```python
from build123d import *

# Parameters (mm, degrees)
ESBO_O1_W                                    = 22.4
ESBO_O1_H                                    = 15
RESSALTO_EXTRUS_O1_DEPTH                     = 2
ESBO_O9_W                                    = 2
ESBO_O9_H                                    = 15
RESSALTO_EXTRUS_O2_DEPTH                     = 1
INCLINA_O2_ANGLE                             = 45
ESBO_O11_W                                   = 2
ESBO_O11_H                                   = 21.213203436
RESSALTO_EXTRUS_O4_DEPTH                     = 22
FILETE1_START                                = 20.4
FILETE1_DEPTH                                = 2
FILETE1_2_DEPTH                              = 22.4
FILETE1_3_DEPTH                              = 2
ESCAREADO_PARA_SFHCS_M31_D                   = 3.4
ESCAREADO_PARA_SFHCS_M31_DEPTH               = 7.5
ESCAREADO_PARA_SFHCS_M31_CSINK_D             = 6.72
ESCAREADO_PARA_SFHCS_M31_CSINK_ANGLE         = 90
ESCAREADO_PARA_SFHCS_M31_TIP                 = 1.021463052
FILETE2_R                                    = 3
ESCAREADO_PARA_PARAFUSO_COM_CABE_A_E_2_COUNT = 2
ESCAREADO_PARA_PARAFUSO_COM_CABE_A_E_2_PITCH = 9


with BuildPart() as part:
    # Esboço1 → Ressalto-extrusão1 (new body)
    with BuildSketch(Plane(origin=(0, 0, 0), x_dir=(1, 0, 0), z_dir=(0, 1, 0))):
        with Locations((11.2, 7.5)):
            Rectangle(ESBO_O1_W, ESBO_O1_H)
    extrude(amount=RESSALTO_EXTRUS_O1_DEPTH)

    # Esboço9 → Ressalto-extrusão2 (add)
    with BuildSketch(Plane.XZ):
        with Locations((21.4, -7.5)):
            Rectangle(ESBO_O9_W, ESBO_O9_H)
    extrude(amount=RESSALTO_EXTRUS_O2_DEPTH)

    # Inclinação2
    inclina_o2_faces = [part.faces().sort_by_distance(p)[0] for p in [
        (21.4, -1, -7.5),
    ]]
    draft(inclina_o2_faces, Plane(origin=(0, 2, 0), x_dir=(1, 0, 0), z_dir=(0, 0, 1)), INCLINA_O2_ANGLE)

    # Esboço11 → Ressalto-extrusão4 (add)
    with BuildSketch(Plane(origin=(0, -0.5, 0.5), x_dir=(1, 0, 0), z_dir=(0, -0.7071067811865462, 0.7071067811865488))):
        with Locations((21.4, -11.313708499)):
            Rectangle(ESBO_O11_W, ESBO_O11_H)
    extrude(amount=RESSALTO_EXTRUS_O4_DEPTH)

    # Filete1: read off the stored shape, not the designer's step
    # Filete1 outline → Filete1 (cut)
    with BuildSketch(Plane.YZ.offset(FILETE1_START)):
        with BuildLine():
            ThreePointArc((-23.627416998, 8.485281374), (-16.556349186, 11.414213562), (-9.485281374, 8.485281374))
            Line((-9.485281374, 8.485281374), (-16.556349186, 15.556349186))
            Line((-16.556349186, 15.556349186), (-23.627416998, 8.485281374))
        make_face()
        with BuildLine():
            Line((-16, -15), (-11.857864376, -15))
            ThreePointArc((-11.857864376, -15), (-15.6846987, -14.238795325), (-18.928932188, -12.071067812))
            Line((-18.928932188, -12.071067812), (-16, -15))
        make_face()
        with BuildLine():
            ThreePointArc((-24.485281374, -6.514718626), (-27.414213562, 0.556349186), (-24.485281374, 7.627416998))
            Line((-24.485281374, 7.627416998), (-31.556349186, 0.556349186))
            Line((-31.556349186, 0.556349186), (-24.485281374, -6.514718626))
        make_face()
    extrude(amount=FILETE1_DEPTH, mode=Mode.SUBTRACT)

    # Filete1 2 outline → Filete1 2 (add)
    with BuildSketch(Plane.YZ):
        with BuildLine():
            Line((0, 0), (2, 0))
            ThreePointArc((2, 0), (0.988246282, 0.177135355), (0, 0.457120724))
            Line((0, 0.457120724), (0, 0))
        make_face()
    extrude(amount=FILETE1_2_DEPTH)

    # Filete1 3 outline → Filete1 3 (add)
    with BuildSketch(Plane.YZ.offset(FILETE1_START)):
        with BuildLine():
            Line((0, 0), (0, 0.457120724))
            ThreePointArc((0, 0.457120724), (-2.065182242, 1.434278965), (-3.854676043, 2.854676043))
            Line((-3.854676043, 2.854676043), (-1, 0))
            Line((-1, 0), (0, 0))
        make_face()
    extrude(amount=FILETE1_3_DEPTH)

    # Escareado para SFHCS M31
    with Locations(Plane(origin=(22.4, 0, 0), x_dir=(0, 0, -1), z_dir=(1, 0, 0))):
        with Locations((3, -6), (11, -14), (3, -22), (-5, -14)):
            CounterSinkHole(ESCAREADO_PARA_SFHCS_M31_D / 2, ESCAREADO_PARA_SFHCS_M31_CSINK_D / 2, depth=ESCAREADO_PARA_SFHCS_M31_DEPTH, counter_sink_angle=ESCAREADO_PARA_SFHCS_M31_CSINK_ANGLE)
            with Locations((0, 0, -(ESCAREADO_PARA_SFHCS_M31_DEPTH + ESCAREADO_PARA_SFHCS_M31_TIP / 2))):  # 118° drill point
                Cone(0, ESCAREADO_PARA_SFHCS_M31_D / 2, ESCAREADO_PARA_SFHCS_M31_TIP, mode=Mode.SUBTRACT)

    # Filete2
    # the kernel refuses this fillet: 3 mm, written as the material it adds along each edge
    with BuildSketch(Plane(origin=(20.4, 0, -15), x_dir=(-1, 0, 0), z_dir=(0, 0, 1))) as filete2_piece_1_section:
        with BuildLine():
            CenterArc((FILETE2_R, FILETE2_R), FILETE2_R, 180, 90)
            Line((0, FILETE2_R), (0, 0))
            Line((0, 0), (FILETE2_R, 0))
        make_face()
    filete2_piece_1 = extrude(amount=22.957120724, mode=Mode.PRIVATE)
    filete2_piece_1 = filete2_piece_1 - Plane(origin=(20.4, 3.216391795, 9.925743967), x_dir=(0, -0.12163917811992071, -0.9925743852962912), z_dir=(-1, 0, 0)) * Cylinder(10.000000115, 58, mode=Mode.PRIVATE)
    add(filete2_piece_1)
    # the kernel refuses this fillet: 3 mm, written as the material it takes off along each edge
    with BuildSketch(Plane(origin=(22.4, 2, 7.5), x_dir=(-1, 0, 0), z_dir=(0, 0, -1))) as filete2_2_piece_1:
        with BuildLine():
            CenterArc((FILETE2_R, -FILETE2_R), FILETE2_R, 90, 90)
            Line((0, -FILETE2_R), (0, 0))
            Line((0, 0), (FILETE2_R, 0))
        make_face()
    extrude(amount=30, mode=Mode.SUBTRACT)

    # Esboço16 → Escareado para parafuso com cabeça escareada elevada de M21 (revolve, cut)
    with BuildSketch(Plane(origin=(4, 0, -7.271439638), x_dir=(0, 0, -1), z_dir=(1, 0, 0))):
        Polygon((0, 0), (0, 2), (1.2, 2), (1.2, 1), (2.2, 0), align=None)
    escareado_para_parafuso_com_cabe_a_escar = revolve(axis=Axis((4, -6.35, -7.271439638), (0, 1, 0)), mode=Mode.SUBTRACT)

    # Escareado para parafuso com cabe_a e 2: Escareado para parafuso com cabeça escareada elevada de M21 ×2
    with Locations(*[(i * ESCAREADO_PARA_PARAFUSO_COM_CABE_A_E_2_PITCH, 0, 0) for i in range(1, ESCAREADO_PARA_PARAFUSO_COM_CABE_A_E_2_COUNT)]):
        add(escareado_para_parafuso_com_cabe_a_escar, mode=Mode.SUBTRACT)


solid = part.part
```
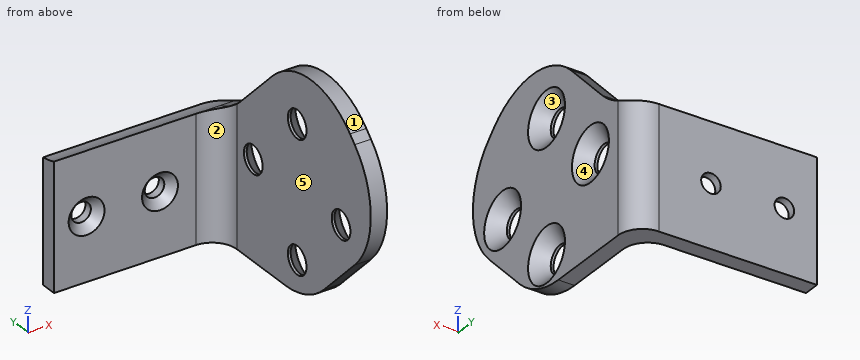
The model under review builds one solid part; all positions refer to its coordinate system, in mm. Face numbers are marked on the shaded views. A direction names the side the tool comes from. Round coordinates to 2 decimals unless told otherwise and drop trailing zeros. Order: outer loops, then holes, each group sorted by start corner. A loop starts at its lowest first (then second) coordinate and runs counter-clockwise, first axis right, second up.
Item 1: Draft analysis for pull direction Z (two halves, no side actions). For the marked faces 1, 2 and 3, state which applies: released by +Z, released by -Z, zero draft, split by the parting line, or undercut.
Working result:
face 1: released by +Z
face 2: zero draft
face 3: undercut
Item 2: To check wall thickness, follow probe 1 along Z at (x, y) = (20.6, -14); probe 2 along X at (y, z) = (-10, 4); probe 3 along Y at (x, z) = (20.55, -3). State the ranges of each line that lie inside material, in increasing order.
Working result:
probe 1: z = -14.77 to -12.7, -9.3 to 3.3, 6.7 to 11.08
probe 2: x = 20.4 to 22.4
probe 3: y = -26.76 to -23.7, -20.3 to -7.7, -4.3 to 1.77
Item 3: Add section D-D, the plane x = 8.25. State the section outline as (y, z) points, and give its area (3 significant figures).
Working result:
outline: (0, -15) - (2, -15) - (2, 0) arc R10 cw to (0, 0.46) - close
area: 30.4 mm2
Item 4: For pin 1 (3 mm diameter, centred on x = 13, z = -7.27, fed in from -Y); pin 2 (10 mm diameter, centred on x = 12, z = -6, fed in from -Y); pin 3 (5 mm diameter, centred on y = -17, z = -4.5, fed in from -X), all flat-tipped, find the tip position at first contact; note any pin that passes through.
Working result:
pin 1: stops at y = 0.7
pin 2: stops at y = 0
pin 3: stops at x = 20.4
Item 5: Add section C-C, the plane y = -6. State the section outline as (x, z) points, and give its area (3 significant figures).
Working result:
outline: (20.4, -15) - (22.4, -15) - (22.4, -6.36) - (20.74, -4.7) - (20.4, -4.7) - close; (20.4, -1.3) - (20.74, -1.3) - (22.4, 0.36) - (22.4, 5) - (20.4, 5) - close
area: 30.4 mm2
Item 6: Machinability: for the marked faces 4 and 5, which of the approach directions +Z, -Z, +X, -X, +Y, -Y give a long, thin tool a straight path to every point of the face, cutting with its end or side? Answer none if there is none.
Working result:
face 4: +X
face 5: +Z, -Z, -X, -Y
Item 7: Add section B-B, the plane x = 4. State the section outline as (y, z) points, and give its area (3 significant figures).
Working result:
outline: (0, -15) - (2, -15) - (2, -8.47) - (1, -8.47) - (0, -9.47) - close; (0, -5.07) - (1, -6.07) - (2, -6.07) - (2, 0) arc R10 cw to (0, 0.46) - close
area: 24.6 mm2
Item 8: Add section A-A, the plane z = -11. State the section outline as (x, y) points.
Working result:
outline: (0, 0) - (17.4, 0) arc R3 cw to (20.4, -3) - (20.4, -12.3) - (20.74, -12.3) - (22.4, -10.64) - (22.4, -1) arc R3 ccw to (19.4, 2) - (0, 2) - close; (20.4, -20) - (22.4, -20) - (22.4, -17.36) - (20.74, -15.7) - (20.4, -15.7) - close
